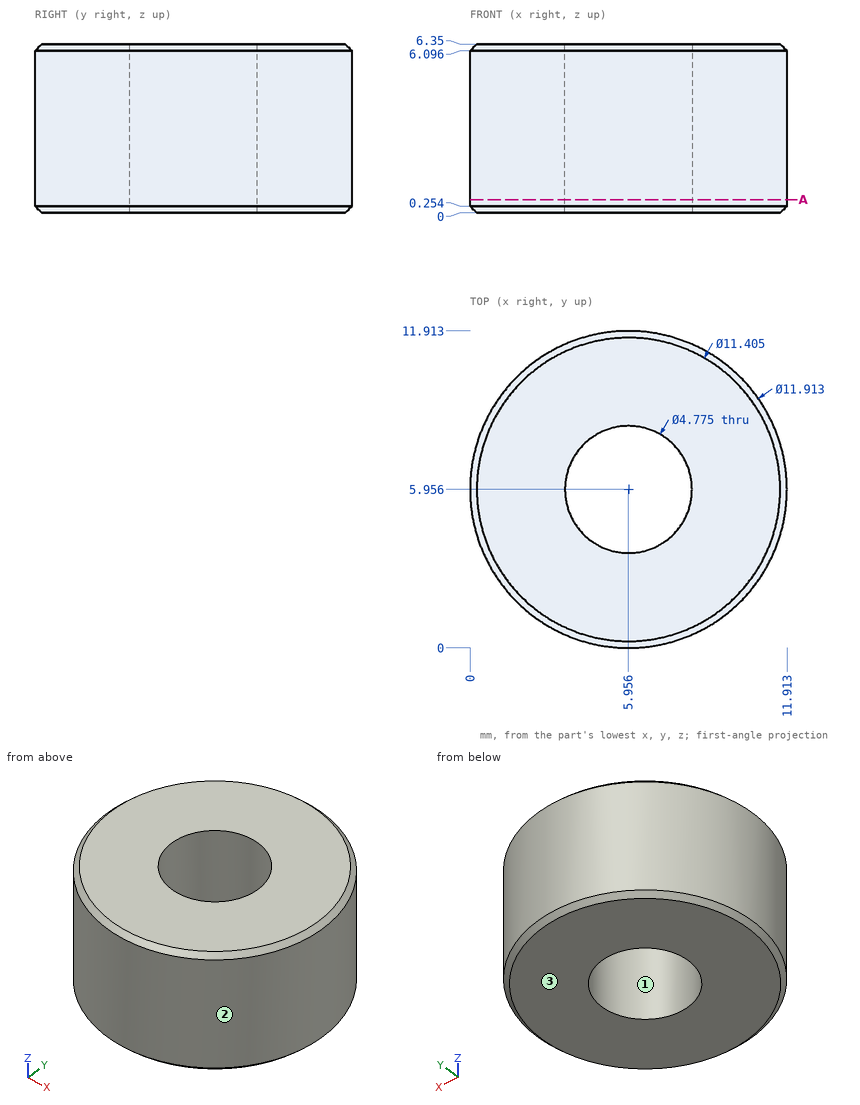
Verification items for this drawing (mm, ordinates from the low corner). Round coordinates to 2 decimals unless told otherwise and drop trailing zeros. Order: outer loops, then holes, each group sorted by start corner. A loop starts at its lowest first (then second) coordinate and runs counter-clockwise, first axis right, second up. Notation, with made-up numbers: (43.5, -9) - (69.5, -9) arc R30 ccw to (69.5, 19) - close; hole circle Ø1 at (83.25, 11.5). An arc over 180 degrees is marked (long way). Use CSV: the item, a comma, the result in double quotes.
(1) Thickness scan on probe 1 along X at (y, z) = (7.5, 5.5) (1 decimal); probe 2 along Y at (x, z) = (6.75, 5) (1 decimal). Record the ranges inside material, lowest first. Write a range as from..to.
Entries:
probe 1,"0.2..4.1, 7.8..11.7"
probe 2,"0.1..3.7, 8.2..11.9"
(2) Section check A-A on z = 0.5. Record the boundary of the cut face in (x, y) (1 decimal).
Entries:
outline,"circle Ø11.9 at (6, 6); hole circle Ø4.8 at (6, 6)"
(3) Gauge pin test, flat ends, axial feed: pin 1 Ø1 at (x, y) = (5, 4) entering from +Z; pin 2 Ø1.5 at (y, z) = (1, 1) entering from -X; pin 3 Ø3 at (y, z) = (2.5, 1) entering from +X. Record the tip position at first contact, or that the pin passes through.
Entries:
pin 1,"z = 6.35"
pin 2,"x = 1.74"
pin 3,"x = 11.58"
(4) Mould release check, pull along Y, two halves, no side actions. Record for the marked faces 1, 2 and 3: released by +Y, released by -Y, zero draft, split by the parting line, or undercut.
Entries:
face 1,"undercut"
face 2,"split by the parting line"
face 3,"zero draft"
